```python
from build123d import *

# Parameters (mm, degrees)
SKETCH1_W             = 158.75
SKETCH1_H             = 107.95
SKETCH1_W_2           = 152.4
SKETCH1_H_2           = 16.134929366
BOSS_EXTRUDE1_DEPTH   = 1.524
CUT_EXTRUDE1_DEPTH    = 2.524
F_6_32_TAPPED_HOLE1_D = 2.7051
F_6_32_TAPPED_HOLE2_D = 2.7051


with BuildPart() as part:
    # Sketch1 → Boss-Extrude1 (new body)
    with BuildSketch(Plane(origin=(0, 0, 0), x_dir=(1, 0, 0), z_dir=(0, 1, 0))):
        Rectangle(SKETCH1_W, SKETCH1_H)
        with BuildLine():
            Line((-76.2, -25.4), (-76.2, -20.767464683))
            Line((-76.2, -20.767464683), (76.2, -20.767464683))
            Line((76.2, -20.767464683), (76.2, -25.4))
            ThreePointArc((76.2, -25.4), (58.239487758, -32.839487758), (50.8, -50.8))
            Line((50.8, -50.8), (-50.8, -50.8))
            ThreePointArc((-50.8, -50.8), (-58.239487758, -32.839487758), (-76.2, -25.4))
        make_face(mode=Mode.SUBTRACT)
        Rectangle(SKETCH1_W_2, SKETCH1_H_2, mode=Mode.SUBTRACT)
        with BuildLine():
            Line((76.2, 20.767464683), (-76.2, 20.767464683))
            Line((-76.2, 20.767464683), (-76.2, 25.4))
            ThreePointArc((-76.2, 25.4), (-58.239487758, 32.839487758), (-50.8, 50.8))
            Line((-50.8, 50.8), (50.8, 50.8))
            ThreePointArc((50.8, 50.8), (58.239487758, 32.839487758), (76.2, 25.4))
            Line((76.2, 25.4), (76.2, 20.767464683))
        make_face(mode=Mode.SUBTRACT)
    extrude(amount=BOSS_EXTRUDE1_DEPTH)

    # Sketch3 → Cut-Extrude1 (cut, through all)
    with BuildSketch(Plane(origin=(0, 1.524, 0), x_dir=(1, 0, 0), z_dir=(0, 1, 0))):
        with BuildLine():
            Line((-60.96, 16.004964683), (60.96, 16.004964683))
            ThreePointArc((60.96, 16.004964683), (62.5475, 14.417464683), (60.96, 12.829964683))
            Line((60.96, 12.829964683), (-60.96, 12.829964683))
            ThreePointArc((-60.96, 12.829964683), (-62.5475, 14.417464683), (-60.96, 16.004964683))
        make_face()
        with BuildLine():
            Line((-60.96, -16.004964683), (60.96, -16.004964683))
            ThreePointArc((60.96, -16.004964683), (62.5475, -14.417464683), (60.96, -12.829964683))
            Line((60.96, -12.829964683), (-60.96, -12.829964683))
            ThreePointArc((-60.96, -12.829964683), (-62.5475, -14.417464683), (-60.96, -16.004964683))
        make_face()
    extrude(amount=-CUT_EXTRUDE1_DEPTH, mode=Mode.SUBTRACT)

    # #6-32 Tapped Hole1 (through all)
    with Locations(Plane(origin=(0, 7.8105, 0), x_dir=(-1, 0, 0), z_dir=(0, 1, 0))):
        with Locations((73.025, -47.625), (73.025, 47.625), (-73.025, 47.625), (-73.025, -47.625)):
            Hole(F_6_32_TAPPED_HOLE1_D / 2)

    # #6-32 Tapped Hole2 (through all)
    with Locations(Plane(origin=(0, 1.524, 0), x_dir=(-1, 0, 0), z_dir=(0, 1, 0))):
        with Locations((73.025, -47.625), (73.025, 47.625), (-73.025, 47.625), (-73.025, -47.625)):
            Hole(F_6_32_TAPPED_HOLE2_D / 2)


solid = part.part
```
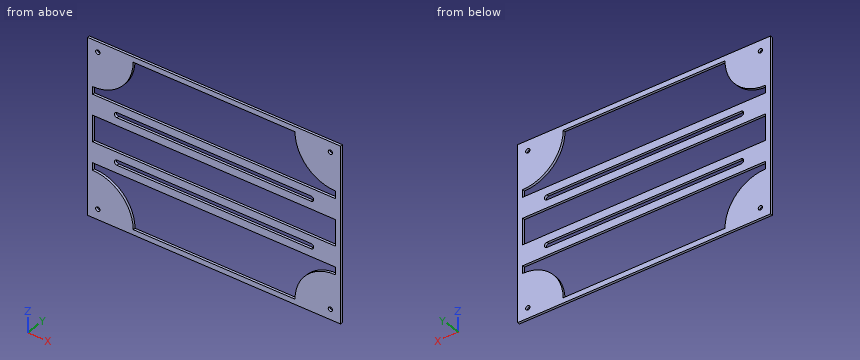
Verification items for the finished model (mm, model axes). Coordinates: 2 decimals unless noted, no trailing zeros. Loops run counter-clockwise (first coordinate to the right, second up) from the corner with the lowest first, then second, coordinate; pieces in that order, holes last. Notation, with made-up numbers: (72.25, 83) -> (122.25, 83) arc R32 ccw to (122.25, 121) -> close; hole circle Ø8 at (31.5, 28). An arc over 180 degrees is marked (long way). Answer in a Markdown table with one row per item.
1) Section check B-B (z = -5). Record the cut outline in (x, y) (3 decimals).
The answers:
| item | result |
|---|---|
| outline | (-79.375, 0) -> (-76.2, 0) -> (-76.2, 1.524) -> (-79.375, 1.524) -> close; (76.2, 0) -> (79.375, 0) -> (79.375, 1.524) -> (76.2, 1.524) -> close |
2) Section check C-C (y = 0.85). Give the number of separate pieces and of enclosed holes in the cut face, and give its area (3 significant figures).
The answers:
| item | result |
|---|---|
| separate pieces | 1 |
| enclosed holes | 9 |
| area | 6,740 mm2 |
3) Depth check by flat-ended pin: P1, Ø5, axis at x = -34, z = 24.5, coming from the +Y side. Enter the tip coordinate at first touch or a pass-through.
The answers:
| item | result |
|---|---|
| P1 | passes through |
4) Section check A-A (x = -47.5). Record the cut outline in (y, z) (3 decimals).
The answers:
| item | result |
|---|---|
| outline | (0, -53.975) -> (1.524, -53.975) -> (1.524, -50.8) -> (0, -50.8) -> close; (0, -20.767) -> (1.524, -20.767) -> (1.524, -16.005) -> (0, -16.005) -> close; (0, -12.83) -> (1.524, -12.83) -> (1.524, -8.067) -> (0, -8.067) -> close; (0, 8.067) -> (1.524, 8.067) -> (1.524, 12.83) -> (0, 12.83) -> close; (0, 16.005) -> (1.524, 16.005) -> (1.524, 20.767) -> (0, 20.767) -> close; (0, 50.8) -> (1.524, 50.8) -> (1.524, 53.975) -> (0, 53.975) -> close |
5) Scan lines: line 1 along Z through (x, y) = (-44, 0.85) (3 decimals); line 2 along X through (y, z) = (0.75, 24) (3 decimals); line 3 along X through (y, z) = (1.3, 48.5) (3 decimals). Record each from-to range of solid material in increasing order. Write a range as from..to.
The answers:
| item | result |
|---|---|
| line 1 | z = -53.975..-50.8, -20.767..-16.005, -12.83..-8.067, 8.067..12.83, 16.005..20.767, 50.8..53.975 |
| line 2 | x = -79.375..-76.2, 76.2..79.375 |
| line 3 | x = -79.375..-74.056, -71.994..-50.904, 50.904..71.994, 74.056..79.375 |
6) Section check D-D (z = -39). Record the cut outline in (x, y) (3 decimals).
The answers:
| item | result |
|---|---|
| outline | (-79.375, 0) -> (-53.707, 0) -> (-53.707, 1.524) -> (-79.375, 1.524) -> close; (53.707, 0) -> (79.375, 0) -> (79.375, 1.524) -> (53.707, 1.524) -> close |
